from build123d import *

# Parameters (mm, degrees)
EXTRUDE_1_DEPTH     = 20
SKETCH_3_R          = 16
EXTRUDE_2_DEPTH     = 8
EXTRUDE_START       = -8
SKETCH_4_R          = 16
EXTRUDE_3_DEPTH     = 8
EXTRUDE_4_DEPTH     = 20
SKETCH_5_W          = 8
SKETCH_5_H          = 20
SKETCH_7_W          = 8
SKETCH_7_H          = 20
SKETCH_10_W         = 8
SKETCH_10_H         = 36
EXTRUDE_5_DEPTH     = 160
CUT_EXTRUDE_3_DEPTH = 160


with BuildPart() as part:
    # Sketch 2 → Extrude 1 (new body)
    with BuildSketch(Plane(origin=(0, 0, 0), x_dir=(1, 0, 0), z_dir=(0, 1, 0))):
        with BuildLine():
            Line((-46, 0), (-46, -20))
            Line((-46, -20), (-38, -20))
            Line((-38, -20), (-38, 0))
            ThreePointArc((-38, 0), (0, 38), (38, 0))
            Line((38, 0), (38, -20))
            Line((38, -20), (46, -20))
            Line((46, -20), (46, 0))
            ThreePointArc((46, 0), (0, 46), (-46, 0))
        make_face()
    extrude(amount=EXTRUDE_1_DEPTH)

    # Sketch 3 → Extrude 2 (add)
    with BuildSketch(Plane.ZY.offset(46)):
        with Locations((20, 0)):
            Circle(SKETCH_3_R)
    extrude(amount=-EXTRUDE_2_DEPTH)

    # Sketch 4 → Extrude 3 (add)
    with BuildSketch(Plane(origin=(46, 0, 0), x_dir=(0, 0, -1), z_dir=(1, 0, 0)).offset(EXTRUDE_START)):
        with Locations((-20, 0)):
            Circle(SKETCH_4_R)
    extrude(amount=EXTRUDE_3_DEPTH)



with BuildPart() as body_2:
    # Sketch 3D_1 → Extrude 4 (new, symmetric)
    with BuildSketch(Plane(origin=(-74, 270, 0), x_dir=(0.9909924304103234, 0, 0.13391789600139506), z_dir=(0, -1, 0))):
        with BuildLine():
            Line((0, 0), (2.67835792, 19.819848608))
            Line((2.67835792, 19.819848608), (10.606297363, 18.74850544))
            Line((10.606297363, 18.74850544), (7.927939443, -1.071343168))
            ThreePointArc((7.927939443, -1.071343168), (64.494858714, -75.315424711), (138.738940257, -18.74850544))
            Line((138.738940257, -18.74850544), (141.417298177, 1.071343168))
            Line((141.417298177, 1.071343168), (149.345237621, 0))
            Line((149.345237621, 0), (146.666879701, -19.819848608))
            ThreePointArc((146.666879701, -19.819848608), (63.423515546, -83.243364154), (0, 0))
        make_face()
    extrude(amount=EXTRUDE_4_DEPTH, both=True)


with BuildPart() as part_1:
    add(part.part)

    add(body_2.part)  # Sweep 1 merges body 2
    # Sweep 1: sweep along a path in Sketch 6
    with BuildLine(Plane.XY.offset(20)) as sweep_1_path:
        Line((46, 20), (74, 250))
    # Sketch 5 → Sweep 1 (sweep)
    with BuildSketch(Plane(origin=(0, 20, 0), x_dir=(1, 0, 0), z_dir=(0, 1, 0))):
        with Locations((42, -10)):
            Rectangle(SKETCH_5_W, SKETCH_5_H)
    sweep(path=sweep_1_path.line)

    # Sweep 2: sweep along a path in Sketch 8
    with BuildLine(Plane.XY.offset(20)) as sweep_2_path:
        Line((-46, 20), (-74, 250))
    # Sketch 7 → Sweep 2 (sweep)
    with BuildSketch(Plane(origin=(0, 20, 0), x_dir=(1, 0, 0), z_dir=(0, 1, 0))):
        with Locations((-42, -10)):
            Rectangle(SKETCH_7_W, SKETCH_7_H)
    sweep(path=sweep_2_path.line)

    # Sketch 10 → Extrude 5 (add)
    with BuildSketch(Plane.XZ.offset(-250)):
        with Locations((-70, 20)):
            Rectangle(SKETCH_10_W, SKETCH_10_H)
    extrude(amount=-EXTRUDE_5_DEPTH)

    # Sketch 12 → Cut-Extrude 3 (cut)
    with BuildSketch(Plane.ZY.offset(74)):
        with BuildLine():
            Line((20, 401), (2, 401))
            Line((2, 401), (2, 419))
            ThreePointArc((2, 419), (32.727922061, 431.727922061), (20, 401))
        make_face()
    extrude(amount=-CUT_EXTRUDE_3_DEPTH, mode=Mode.SUBTRACT)


solid = part_1.part
For this review, take the finished solid that the model builds, in its own axes (mm). A direction names the side the tool comes from. Round coordinates to 2 decimals unless told otherwise and drop trailing zeros. Loops run counter-clockwise (first coordinate to the right, second up) from the corner with the lowest first, then second, coordinate; pieces in that order, holes last. Notation, with made-up numbers: (4.5, 64) - (53.5, 64) arc R24 cw to (53.5, 79) - close; hole circle Ø5 at (71, 25.25). An arc over 180 degrees is marked (long way). Put each result on its own line as item: value. Start each with the question number.
1. Consider section B-B on y = 230.5. State the section outline as (x, z) points, plus the area to 3 significant figures.
2. Consider section C-C on x = -16. State the section outline as (y, z) points.
3. For faces 1 (the flat face through (66, 270, 10)), 2 (the flat face through (56, 144, 0)), 3 (the flat face through (3.2, 20, -38.4)), list the 3-axis set-ups (+Z, -Z, +X, -X, +Y, -Y) from which the entire face can be reached by the end or side of a thin tool; tool diameter is ignored.
4. Consider section A-A on z = 15. State the section outline as (x, y) points, plus the area to 3 significant figures.
5. Insertion check: P1, Ø11, axis at x = 56.5, y = 177.5, coming from the +Z side; P2, Ø18, axis at y = -6.5, z = 21, coming from the -X side; P3, Ø5, axis at y = 257.5, z = -20, coming from the +X side; P4, Ø25, axis at x = -23, z = -10.5, coming from the -Y side. Each pin has a flat end and moves straight along its axis. Give the tip position at first contact, or say it passes through.
6. Mouldability with a two-part tool opening along X and no side actions: class faces 4 (the flat face through (-46, 2, 18)), 5 (the cylindrical face through (-70.056, 403.478, 29.114)), 6 (the flat face through (52.196, 136.61, 9.86)) as +X half, -X half, draft (parallel to the pull), parting line (faces both ways), or undercut.
7. Consider section D-D on z = -20.5. State the section outline as (x, y) points.
8. For probe 1 along Y at (x, z) = (-42, -58); probe 2 along X at (y, z) = (10, -5); probe 3 along X at (y, z) = (99, 13.5), list the stretches that pass through material, from the lowest coordinate up. Write a range as [from, to].
Result sheet:
1. outline: (-71.63, 0) - (-63.63, 0) - (-63.63, 20) - (-71.63, 20) - close; (63.63, 0) - (71.63, 0) - (71.63, 20) - (63.63, 20) - close
1. area: 320 mm^2
2. outline: (0, -43.13) - (20, -43.13) - (20, -34.47) - (0, -34.47) - close; (250, -72.25) - (290, -72.25) - (290, -64.03) - (250, -64.03) - close
3. face 1: +Z, +Y
3. face 2: -Z, +X, -X
3. face 3: -Z, +X, -X, +Y
4. outline: (-74, 250) - (-46, 20) - (-46, -15.2) - (-38, -15.2) - (-38, 20) - (-66, 250) - (-66, 401) - (-74, 401) - close; (38, -15.2) - (46, -15.2) - (46, 20) - (74, 250) - (74, 290) - (66, 290) - (66, 250) - (38, 20) - close
4. area: 5,770 mm^2
5. P1: z = 20
5. P2: x = -46
5. P3: x = 71.9
5. P4: through
6. face 4: -X half
6. face 5: draft
6. face 6: undercut
7. outline: (-71.1, 250) - (-62.74, 250) - (-62.74, 290) - (-71.1, 290) - close; (-41.18, 0) - (-32, 0) - (-32, 20) - (-41.18, 20) - close; (32, 0) - (41.18, 0) - (41.18, 20) - (32, 20) - close; (62.74, 250) - (71.1, 250) - (71.1, 290) - (62.74, 290) - close
8. probe 1: [250, 290]
8. probe 2: [-45.73, -37.67], [37.67, 45.73]
8. probe 3: [-55.62, -47.62], [47.62, 55.62]
